Part model, mm, in its own coordinate system. A direction names the side the tool comes from. Round coordinates to 2 decimals unless told otherwise and drop trailing zeros. Loops run counter-clockwise (first coordinate to the right, second up) from the corner with the lowest first, then second, coordinate; pieces in that order, holes last.
from build123d import *

# Parameters (mm, degrees)
F0_R     = 50
F0_R_2   = 3.175
F0_R_3   = 25
F1_DEPTH = 12.7
F2_W     = 9.525
F2_H     = 76
F3_DEPTH = 37
F4_R     = 1.6
F5_DEPTH = 83.001
F6_SIZE  = 5


# Not quite as in the source:
# - a feature names something its author has since deleted; it is built from what else it names


with BuildPart() as f1:
    # F0 (on Front) → F1 (new body)
    with BuildSketch(Plane.XZ):
        Circle(F0_R)
        with Locations((-15.7401153702, -38)):
            Circle(F0_R_2, mode=Mode.SUBTRACT)
        with Locations((-38, -15.7401153702)):
            Circle(F0_R_2, mode=Mode.SUBTRACT)
        with Locations((15.7401153702, -38)):
            Circle(F0_R_2, mode=Mode.SUBTRACT)
        with Locations((38, -15.7401153702)):
            Circle(F0_R_2, mode=Mode.SUBTRACT)
        with Locations((-38, 15.7401153702)):
            Circle(F0_R_2, mode=Mode.SUBTRACT)
        with Locations((-15.7401153702, 38)):
            Circle(F0_R_2, mode=Mode.SUBTRACT)
        Circle(F0_R_3, mode=Mode.SUBTRACT)
        with Locations((38, 15.7401153702)):
            Circle(F0_R_2, mode=Mode.SUBTRACT)
        with Locations((15.7401153702, 38)):
            Circle(F0_R_2, mode=Mode.SUBTRACT)
    extrude(amount=F1_DEPTH)

    # F2 (on face) → F3 (join)
    with BuildSketch(Plane.XZ.offset(12.7)):
        with Locations((-28.2375, 0)):
            Rectangle(F2_W, F2_H)
        with Locations((28.2375, 0)):
            Rectangle(F2_W, F2_H)
    extrude(amount=F3_DEPTH)

    # F4 (on face) → F5 (cut, through all)
    with BuildSketch(Plane(origin=(-33, 0, 0), x_dir=(0, -1, 0), z_dir=(-1, 0, 0))):
        with Locations((32.7, 30)):
            Circle(F4_R)
        with Locations((32.7, 10)):
            Circle(F4_R)
        with Locations((32.7, -10)):
            Circle(F4_R)
        with Locations((32.7, -30)):
            Circle(F4_R)
    extrude(amount=-F5_DEPTH, mode=Mode.SUBTRACT)

    # F6
    f6_edges = [f1.edges().sort_by_distance(p)[0] for p in [
        (-28.2375, -49.7, -38),
        (28.2375, -49.7, -38),
        (-28.2375, -49.7, 38),
        (28.2375, -49.7, 38),
    ]]
    chamfer(f6_edges, length=F6_SIZE)


solid = f1.part
1) Drop flat-ended pins along their axis: pin 1 Ø8 at (y, z) = (-7, -11) entering from -X; pin 2 Ø12 at (x, y) = (37.5, -38.5) entering from -Z; pin 3 Ø0.5 at (x, z) = (-32.5, 38) entering from +Y; pin 4 Ø1 at (y, z) = (-44, -27.5) entering from +X. Give the stop position or say it passes through.
Values:
pin 1: stops at x = -49.51
pin 2: stops at z = -38
pin 3: stops at y = 0
pin 4: stops at x = 33
2) Tool access for faces 5 (the face through (23.846, -6.261, 7.509)), 6 (the face through (28.2, -47.2, -35.5)), 7 (the face through (39, -12.7, 1)), 8 (the face through (-40, -12.7, 1)), 9 (the face through (28, -49.7, 0)): list every direction of +Z, -Z, +X, -X, +Y, -Y with a clear straight run to the whole face (end or side of a thin tool).
Values:
face 5: +Y
face 6: -Z, +X, -X, -Y
face 7: +Z, -Z, +X, -Y
face 8: +Z, -Z, -X, -Y
face 9: +Z, -Z, +X, -X, -Y
3) Slice it at A-A, the plane z = 30. Give the cut face in (x, y) (3 decimals), then the cut area to 3 significant figures.
Values:
outline: (-40, -12.7) - (-33, -12.7) - (-33, -31.1) - (-23.475, -31.1) - (-23.475, -12.7) - (23.475, -12.7) - (23.475, -31.1) - (33, -31.1) - (33, -12.7) - (40, -12.7) - (40, 0) - (-40, 0) - close; (-33, -49.7) - (-23.475, -49.7) - (-23.475, -34.3) - (-33, -34.3) - close; (23.475, -49.7) - (33, -49.7) - (33, -34.3) - (23.475, -34.3) - close
area: 1,660 mm2
4) Wall check: line 1 along X through (y, z) = (-40, 12.5) (3 decimals); line 2 along Z through (x, y) = (38, -9); line 3 along Z through (x, y) = (-15.5, -5). Give the ranges that are in metal, low to high.
Values:
line 1: x = -33 to -23.475, 23.475 to 33
line 2: z = -32.5 to -18.92, -12.57 to 12.57, 18.92 to 32.5
line 3: z = -47.54 to -41.17, -34.83 to -19.62, 19.62 to 34.83, 41.17 to 47.54
5) Mould opens along X. For faces 1 (the face through (47.69, -6.26, 15.02)), 2 (the face through (23.475, -31, -1)), 3 (the face through (28, -28, 38)), 4 (the face through (33, -31, -1)) say: released by +X, released by -X, zero draft, split by the parting line, or undercut.
Values:
face 1: split by the parting line
face 2: undercut
face 3: zero draft
face 4: released by +X
6) Slice it at C-C, the plane x = 0. Give the cut face in (y, z).
Values:
outline: (-12.7, -50) - (0, -50) - (0, -25) - (-12.7, -25) - close; (-12.7, 25) - (0, 25) - (0, 50) - (-12.7, 50) - close
7) Slice it at B-B, the plane y = -46. Give the cut face in (x, z) (3 decimals).
Values:
outline: (-33, -36.7) - (-23.475, -36.7) - (-23.475, 36.7) - (-33, 36.7) - close; (23.475, -36.7) - (33, -36.7) - (33, 36.7) - (23.475, 36.7) - close
8) Slice it at D-D, the plane x = -38. Give the cut face in (y, z), then the cut area to 3 significant figures.
Values:
outline: (-12.7, -32.5) - (0, -32.5) - (0, -18.92) - (-12.7, -18.92) - close; (-12.7, -12.57) - (0, -12.57) - (0, 12.57) - (-12.7, 12.57) - close; (-12.7, 18.92) - (0, 18.92) - (0, 32.5) - (-12.7, 32.5) - close
area: 664 mm2
